from build123d import *

# Parameters (mm, degrees)
SKETCH1_W           = 20
SKETCH1_H           = 10
SKETCH1_R           = 1.25
BOSS_EXTRUDE1_DEPTH = 6.4
BOSS_EXTRUDE2_START = 1.5
SKETCH1_3_W         = 0.2
SKETCH1_3_H         = 4
BOSS_EXTRUDE2_DEPTH = 3.4
CHAMFER2_SIZE       = 0.5
SKETCH3_R           = 0.75
CUT_EXTRUDE2_DEPTH  = 20.4


with BuildPart() as part:
    # Sketch1 → Boss-Extrude1 (new body)
    with BuildSketch(Plane(origin=(0, 0, 0), x_dir=(1, 0, 0), z_dir=(0, 1, 0))):
        Rectangle(SKETCH1_W, SKETCH1_H)
        with Locations(Location((4.75, -2, 0), (0, 0, 270))):
            Circle(SKETCH1_R, mode=Mode.SUBTRACT)
        with Locations(Location((-4.75, -2, 0), (0, 0, 270))):
            Circle(SKETCH1_R, mode=Mode.SUBTRACT)
    extrude(amount=BOSS_EXTRUDE1_DEPTH)

    # Sketch1_3 → Boss-Extrude2 (add)
    with BuildSketch(Plane(origin=(0, 0, 0), x_dir=(1, 0, 0), z_dir=(0, 1, 0)).offset(BOSS_EXTRUDE2_START)):
        Polygon((7.1, 5), (7.3, 5), (7.3, 5.5), (-7.687995196, 10.5), (-7.751286335, 10.310278542), (7.1, 5.355884662), align=None)
        with BuildLine():
            Line((2.5, 5), (4.5, 5))
            Line((4.5, 5), (4.5, 5.5))
            ThreePointArc((4.5, 5.5), (3.5, 6.5), (2.5, 5.5))
            Line((2.5, 5.5), (2.5, 5))
        make_face()
        with Locations((7.5, -7)):
            Rectangle(SKETCH1_3_W, SKETCH1_3_H)
        with Locations((0, -7)):
            Rectangle(SKETCH1_3_W, SKETCH1_3_H)
        with Locations((-7.5, -7)):
            Rectangle(SKETCH1_3_W, SKETCH1_3_H)
    extrude(amount=BOSS_EXTRUDE2_DEPTH)

    # Chamfer2
    chamfer2_edges = [part.edges().sort_by_distance(p)[0] for p in [
        (-7.5, 1.5, 9),
        (-7.5, 4.9, 9),
        (0, 1.5, 9),
        (0, 4.9, 9),
        (7.5, 4.9, 9),
        (7.5, 1.5, 9),
    ]]
    chamfer(chamfer2_edges, length=CHAMFER2_SIZE)

    # Sketch3 → Cut-Extrude2 (cut)
    with BuildSketch(Plane.ZY.offset(7.6)):
        with Locations((7.75, 3.2)):
            Circle(SKETCH3_R)
    extrude(amount=-CUT_EXTRUDE2_DEPTH, mode=Mode.SUBTRACT)


solid = part.part
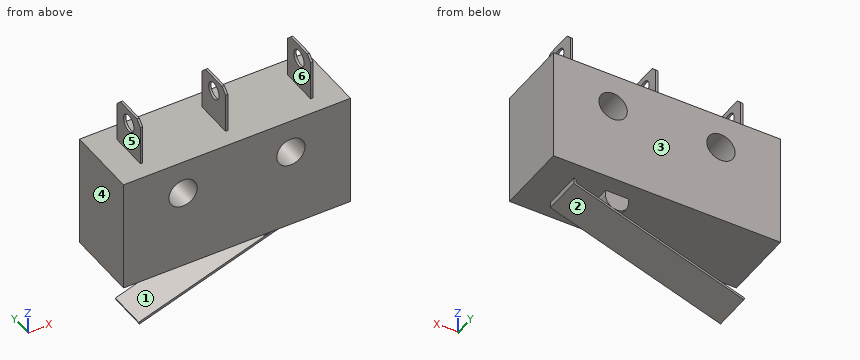
Could you check a few things on this model? Use its own coordinates, in mm. Face numbers are marked on the shaded views. A direction names the side the tool comes from. Give positions to 0.01 mm unless a question says otherwise; leave off trailing zeros. Order: outer loops, then holes, each group sorted by start corner. A loop starts at its lowest first (then second) coordinate and runs counter-clockwise, first axis right, second up. Notation, with made-up numbers: (-25.5, 6) -> (-6.5, 6) arc R14 cw to (-6.5, 20) -> close; hole circle Ø3 at (44, -6). An arc over 180 degrees is marked (long way). Return JSON: item names as keys, results as strings.
1. On a 3-axis mill with a long thin cutter (end or side, diameter ignored), from which of +Z, -Z, +X, -X, +Y, -Y can I reach the whole of each face in a straight line? I mean the marked faces 4, 5 and 6. Say none if no direction works.
Answer list:
{"face 4": "+Z, -Z, -X, +Y, -Y", "face 5": "+Z, -X, +Y, -Y", "face 6": "+Z, +Y, -Y"}
2. Imagine slicing it at D-D on y = 3.2. Give the number of separate pieces and of enclosed holes in the cut face, then the cut area to 3 significant figures.
Answer list:
{"separate pieces": "4", "enclosed holes": "2", "area": "197 mm2"}
3. Imagine slicing it at C-C on x = -5.25. List the corners of the cut face in (y, z) for me.
Answer list:
{"outline": "(0, -5) -> (6.4, -5) -> (6.4, 0.85) -> (0, 0.85) -> close; (0, 3.15) -> (6.4, 3.15) -> (6.4, 5) -> (0, 5) -> close; (1.5, -9.69) -> (4.9, -9.69) -> (4.9, -9.48) -> (1.5, -9.48) -> close"}
4. I need wall thicknesses on line 1 (X direction, y = 3.25, z = 2); line 2 (X direction, y = 2, z = 5.25); line 3 (Y direction, x = 7.55, z = 7.75). Which ranges of each line are inside material? Lowest first, please. Write a range as from..to.
Answer list:
{"line 1": "x = -10..-6, -3.5..3.5, 6..10", "line 2": "x = -7.6..-7.4, -0.1..0.1, 7.4..7.6", "line 3": "y = 1.5..2.45, 3.95..4.9"}
5. Imagine slicing it at A-A on z = 7.75. List the corners of the cut face in (x, y) for me.
Answer list:
{"outline": "(-7.6, 1.5) -> (-7.4, 1.5) -> (-7.4, 2.45) -> (-7.6, 2.45) -> close; (-7.6, 3.95) -> (-7.4, 3.95) -> (-7.4, 4.9) -> (-7.6, 4.9) -> close; (-0.1, 1.5) -> (0.1, 1.5) -> (0.1, 2.45) -> (-0.1, 2.45) -> close; (-0.1, 3.95) -> (0.1, 3.95) -> (0.1, 4.9) -> (-0.1, 4.9) -> close; (7.4, 1.5) -> (7.6, 1.5) -> (7.6, 2.45) -> (7.4, 2.45) -> close; (7.4, 3.95) -> (7.6, 3.95) -> (7.6, 4.9) -> (7.4, 4.9) -> close"}
6. Thinking about a two-plate mould opening in Z: for the marked faces 1, 2 and 3, which applies, pulls with the +Z half, pulls with the -Z half, needs draft (parallel to the pull), parting line crosses it, or undercut?
Answer list:
{"face 1": "undercut", "face 2": "pulls with the -Z half", "face 3": "needs draft"}
7. Imagine slicing it at B-B on y = 0.5. List the corners of the cut face in (x, z) for me, then the cut area to 3 significant figures.
Answer list:
{"outline": "(-10, -5) -> (10, -5) -> (10, 5) -> (-10, 5) -> close; hole circle Ø2.5 at (-4.75, 2); hole circle Ø2.5 at (4.75, 2)", "area": "190 mm2"}
8. For pin 1 Ø2.5 at (y, z) = (3.2, 7.75) entering from +X; pin 2 Ø3 at (x, z) = (0, -8) entering from +Y; pin 3 Ø3 at (x, y) = (-3, 3) entering from -Z; pin 4 Ø1.4 at (y, z) = (3.2, 7.75) entering from +X, each with a flat end and sliding along its axis, tell me the tip position at first contact or that it passes through.
Answer list:
{"pin 1": "stops at x = 7.6", "pin 2": "stops at y = 4.9", "pin 3": "stops at z = -9.44", "pin 4": "passes through"}
